Input: part model. Units: mm. Frame: model coordinates. Coordinates: 2 decimals unless noted, no trailing zeros. Write each loop counter-clockwise with the first axis right and the second up, starting at its lowest first coordinate (ties: lowest second). Pieces come first, ordered by that corner, then holes.
1) Draft query along X for faces 1 (the flat face through (90, 1, -1)), 2 (the cylindrical face through (-77.217, 1.479, 25.919)), 3 (the flat face through (1, 1, 37.5)). Return one class per face: pulls with the +X half, pulls with the -X half, needs draft (parallel to the pull), parting line crosses it, or undercut.
2) Section query A-A (x = -75). Output: boundary loops of the cut face in (y, z), then the cut area to 3 significant figures.
3) Line query: L1, parallel to Z at x = 75, y = 1.9. Output: solid intervals per line, ascending.
4) Pin query (flat end, axial travel): pin 1 Ø2 at (x, z) = (-71.5, 28) entering from -Y. Return the tip coordinate at first contact, or that it passes through.
5) Section query B-B (z = -25). Output: boundary loops of the cut face in (x, y).
Autodesk Inventor part; units mm, degrees
ref_plane "YZ Plane" through (0, 0, 0) normal (1, 0, 0) x (0, 1, 0)
ref_plane "XZ Plane" through (0, 0, 0) normal (0, 1, 0) x (-1, 0, 0)
ref_plane "XY Plane" through (0, 0, 0) normal (0, 0, 1) x (1, 0, 0)
sketch "Sketch1" plane through (0, 0, 0) normal (0, 1, 0) x (-1, 0, 0)
  line L0 (-90, 37.5) -> (90, 37.5)
  line L1 (90, 37.5) -> (90, -37.5)
  line L2 (90, -37.5) -> (-90, -37.5)
  line L3 (-90, -37.5) -> (-90, 37.5)
  line L4 (-90, 37.5) -> (90, -37.5) construction
  line L5 (90, 37.5) -> (-90, -37.5) construction
  point P0 (0, 0)
  dimension "d0" = 180
  dimension "d1" = 75
extrude "Extrusion1" add sketch "Sketch1" along normal blind 3
sketch "Sketch2" plane through (0, 0, 0) normal (0, -1, 0) x (1, 0, 0)
  circle A0 centre (75, 25) radius 2.4
  circle A1 centre (75, -25) radius 2.4
  circle A2 centre (97.5, 25) radius 2.7
  circle A3 centre (97.5, -25) radius 2.7
  line L0 (90, 37.5) -> (90, -37.5)
  point P0 (0, 0)
  dimension "d4" = 4.8
  dimension "d5" = 15
ref_plane "Work Plane1" through (0, 0, 37.5) normal (1, 0, 0) x (0, 0, -1)
extrude "Extrusion2" cut sketch "Sketch2" against normal through all contours A0 | A1
mirror "Mirror1" about plane through (0, 0, 37.5) normal (1, 0, 0) of "Extrusion2"
properties part number "Side Plane" material "Wood (Birch)"
Answer:
1. face 1: pulls with the +X half
1. face 2: undercut
1. face 3: needs draft
2. outline: (0, -37.5) - (3, -37.5) - (3, -27.4) - (0, -27.4) - close; (0, -22.6) - (3, -22.6) - (3, 22.6) - (0, 22.6) - close; (0, 27.4) - (3, 27.4) - (3, 37.5) - (0, 37.5) - close
2. area: 196 mm2
3. L1: z = -37.5 to -27.4, -22.6 to 22.6, 27.4 to 37.5
4. pin 1: stops at y = 0
5. outline: (-90, 0) - (-77.4, 0) - (-77.4, 3) - (-90, 3) - close; (-72.6, 0) - (72.6, 0) - (72.6, 3) - (-72.6, 3) - close; (77.4, 0) - (90, 0) - (90, 3) - (77.4, 3) - close
